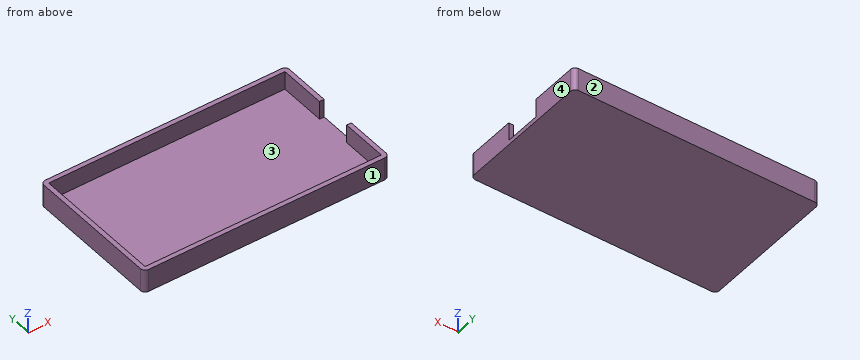
```python
from build123d import *

# Parameters (mm, degrees)
SKETCH_W      = 53.5
SKETCH_H      = 30.46
PAD_DEPTH     = 1
SKETCH001_W   = 53.5
SKETCH001_H   = 30.46
SKETCH001_W_2 = 51.5
SKETCH001_H_2 = 28.46
PAD001_DEPTH  = 4
SKETCH002_W   = 8
SKETCH002_H   = 4
POCKET_DEPTH  = 1
FILLET_R      = 1


with BuildPart() as part:
    # Sketch → Pad (new body)
    with BuildSketch(Plane.XY):
        Rectangle(SKETCH_W, SKETCH_H)
    extrude(amount=PAD_DEPTH)

    # Sketch001 (on Face6 of Pad) → Pad001 (join)
    with BuildSketch(Plane.XY.offset(1)):
        Rectangle(SKETCH001_W, SKETCH001_H)
        Rectangle(SKETCH001_W_2, SKETCH001_H_2, mode=Mode.SUBTRACT)
    extrude(amount=PAD001_DEPTH)

    # Sketch002 (on Face8 of Pad001) → Pocket (cut)
    with BuildSketch(Plane.YZ.offset(26.75)):
        with Locations((0, 3)):
            Rectangle(SKETCH002_W, SKETCH002_H)
    extrude(amount=-POCKET_DEPTH, mode=Mode.SUBTRACT)

    # Fillet
    fillet_edges = [part.edges().sort_by_distance(p)[0] for p in [
        (26.75, -15.23, 0.5),
        (26.75, -15.23, 3),
        (26.75, 15.23, 3),
        (26.75, 15.23, 0.5),
        (-26.75, 15.23, 3),
        (-26.75, 15.23, 0.5),
        (-26.75, -15.23, 3),
        (-26.75, -15.23, 0.5),
    ]]
    fillet(fillet_edges, radius=FILLET_R)


solid = part.part
```
For this review, take the finished solid that the model builds, in its own axes (mm). Face numbers are marked on the shaded views. Round coordinates to 2 decimals unless told otherwise and drop trailing zeros. Loops run counter-clockwise (first coordinate to the right, second up) from the corner with the lowest first, then second, coordinate; pieces in that order, holes last.
Q1. To check wall thickness, follow line 1 along X through (y, z) = (-6, 1.6); line 2 along Y through (x, z) = (20, 1.75); line 3 along X through (y, z) = (2.5, 1.85). State the ranges of each line that lie inside material, in increasing order.
Result sheet:
line 1: x = -26.75 to -25.75, 25.75 to 26.75
line 2: y = -15.23 to -14.23, 14.23 to 15.23
line 3: x = -26.75 to -25.75
Q2. Add section B-B on x = 20. Write out the cut boundary in (y, z).
Result sheet:
outline: (-15.23, 0) - (15.23, 0) - (15.23, 5) - (14.23, 5) - (14.23, 1) - (-14.23, 1) - (-14.23, 5) - (-15.23, 5) - close
Q3. Mouldability with a two-part tool opening along Y and no side actions: class the marked faces 1, 2, 3 and 4 as +Y half, -Y half, draft (parallel to the pull), parting line (faces both ways), or undercut.
Result sheet:
face 1: -Y half
face 2: +Y half
face 3: undercut
face 4: draft
Q4. Add section A-A on z = 2.9. Write out the cut boundary in (x, y), plus the area to 3 significant figures.
Result sheet:
outline: (-26.75, -14.23) arc R1 ccw to (-25.75, -15.23) - (25.75, -15.23) arc R1 ccw to (26.75, -14.23) - (26.75, -4) - (25.75, -4) - (25.75, -14.23) - (-25.75, -14.23) - (-25.75, 14.23) - (25.75, 14.23) - (25.75, 4) - (26.75, 4) - (26.75, 14.23) arc R1 ccw to (25.75, 15.23) - (-25.75, 15.23) arc R1 ccw to (-26.75, 14.23) - close
area: 155 mm2
Q5. Add section C-C on y = 3.5. Write out the cut boundary in (x, z).
Result sheet:
outline: (-26.75, 0) - (26.75, 0) - (26.75, 1) - (-25.75, 1) - (-25.75, 5) - (-26.75, 5) - close
Q6. Add section D-D on y = 7.5. Write out the cut boundary in (x, z).
Result sheet:
outline: (-26.75, 0) - (26.75, 0) - (26.75, 5) - (25.75, 5) - (25.75, 1) - (-25.75, 1) - (-25.75, 5) - (-26.75, 5) - close
Q7. Insertion check: pin 1 Ø5 at (x, y) = (5, 7) entering from +Z. The pin has a flat end and moves straight along its axis. Give the tip position at first contact, or say it passes through.
Result sheet:
pin 1: stops at z = 1
